Source: three-view drawing plus pictorial views. Frame: mm from the lowest corner of the part. A direction names the side the tool comes from. Give positions to 0.01 mm unless a question says otherwise; leave off trailing zeros. Loops run counter-clockwise (first coordinate to the right, second up) from the corner with the lowest first, then second, coordinate; pieces in that order, holes last. Notation, with made-up numbers: (72, 62.25) -> (107, 62.25) arc R23 cw to (107, 83.25) -> close; hole circle Ø4 at (40, 43.25). An arc over 180 degrees is marked (long way). Put each result on its own line as item: value.
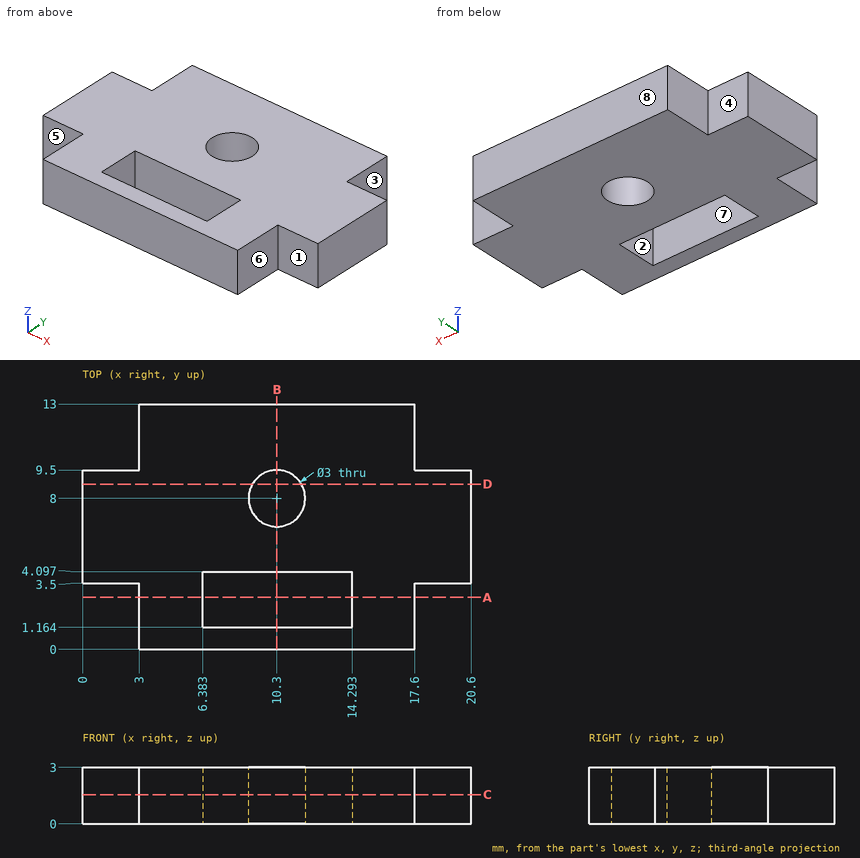
(1) Reachability of the marked faces 1, 2, 3 and 4 from +Z, -Z, +X, -X, +Y, -Y: full face, straight path, thin tool, end or side. Return the list, or none.
Calculated:
face 1: +Z, -Z, +X, -Y
face 2: +Z, -Z
face 3: +Z, -Z, +X, +Y
face 4: +Z, -Z, -X, +Y
(2) Section D-D on y = 8.75. Return loops of the section in (x, z).
Calculated:
outline: (0, 0) -> (9, 0) -> (9, 3) -> (0, 3) -> close; (11.6, 0) -> (20.6, 0) -> (20.6, 3) -> (11.6, 3) -> close
(3) Draft query along Y for the marked faces 5, 6, 7 and 8. Return one class per face: released by +Y, released by -Y, zero draft, split by the parting line, or undercut.
Calculated:
face 5: released by -Y
face 6: zero draft
face 7: undercut
face 8: released by +Y
(4) Line query: probe 1 along Y at (x, z) = (10.3, 1.75); probe 2 along X at (y, z) = (1.5, 1.2); probe 3 along X at (y, z) = (12.5, 1.45). Output: solid intervals per line, ascending. Write a range as from..to.
Calculated:
probe 1: y = 0..1.16, 4.1..6.5, 9.5..13
probe 2: x = 3..6.38, 14.29..17.6
probe 3: x = 3..17.6
(5) First-contact query: P1, Ø0.9, axis at y = 12, z = 2, coming from the -X side; P2, Ø0.9, axis at y = 10.5, z = 1, coming from the +X side; P3, Ø1.5, axis at x = 19, z = 2, coming from the -Y side. Flat tips, straight axial feed; report the tip coordinate or a pass-through.
Calculated:
P1: stops at x = 3
P2: stops at x = 17.6
P3: stops at y = 3.5
(6) Section C-C on z = 1.55. Return loops of the section in (x, y).
Calculated:
outline: (0, 3.5) -> (3, 3.5) -> (3, 0) -> (17.6, 0) -> (17.6, 3.5) -> (20.6, 3.5) -> (20.6, 9.5) -> (17.6, 9.5) -> (17.6, 13) -> (3, 13) -> (3, 9.5) -> (0, 9.5) -> close; hole (6.38, 1.16) -> (14.29, 1.16) -> (14.29, 4.1) -> (6.38, 4.1) -> close; hole circle Ø3 at (10.3, 8)
(7) Section B-B on x = 10.3. Return loops of the section in (y, z).
Calculated:
outline: (0, 0) -> (1.16, 0) -> (1.16, 3) -> (0, 3) -> close; (4.1, 0) -> (6.5, 0) -> (6.5, 3) -> (4.1, 3) -> close; (9.5, 0) -> (13, 0) -> (13, 3) -> (9.5, 3) -> close
(8) Section A-A on y = 2.75. Return loops of the section in (x, z).
Calculated:
outline: (3, 0) -> (6.38, 0) -> (6.38, 3) -> (3, 3) -> close; (14.29, 0) -> (17.6, 0) -> (17.6, 3) -> (14.29, 3) -> close
